```python
from build123d import *

# Parameters (mm, degrees)
SKETCH1_W           = 20.32
SKETCH1_H           = 134.62
BOSS_EXTRUDE1_DEPTH = 2.999994
BOSS_EXTRUDE2_DEPTH = 2.999994
BOSS_EXTRUDE3_DEPTH = 22.86
SKETCH4_R           = 2.54
CUT_EXTRUDE1_DEPTH  = 37.477194


with BuildPart() as part:
    # Sketch1 → Boss-Extrude1 (new body)
    with BuildSketch(Plane.XY):
        with Locations((-1.678928241, 0)):
            Rectangle(SKETCH1_W, SKETCH1_H)
    extrude(amount=BOSS_EXTRUDE1_DEPTH)

    # Sketch2 → Boss-Extrude2 (add)
    with BuildSketch(Plane(origin=(0, -67.31, 0), x_dir=(1, 0, 0), z_dir=(0, 1, 0))):
        Polygon((-11.838928241, 0), (-11.838928241, 16.7386), (8.478742997, 16.7386), (8.481071759, 0), (8.478742997, -2.999994), (8.481071759, -19.738594), (-11.838928241, -19.738594), (-11.838928241, -2.999994), align=None)
    extrude(amount=BOSS_EXTRUDE2_DEPTH)

    # Sketch3 → Boss-Extrude3 (add)
    with BuildSketch(Plane(origin=(0, -67.31, 0), x_dir=(-1, 0, 0), z_dir=(0, -1, 0))):
        Polygon((11.838928241, 16.7386), (11.838928241, 13.72362), (-8.479162457, 13.72362), (-8.478742997, 16.7386), align=None)
        Polygon((-8.481065309, -16.677248459), (-8.481065309, -19.692228459), (11.837025389, -19.692228459), (11.836605929, -16.677248459), align=None)
    extrude(amount=BOSS_EXTRUDE3_DEPTH)

    # Sketch4 → Cut-Extrude1 (cut, through all)
    with BuildSketch(Plane(origin=(0, 0, -16.7386), x_dir=(-1, 0, 0), z_dir=(0, 0, -1))):
        with Locations((1.680092622, -84.961272754)):
            Circle(SKETCH4_R)
    extrude(amount=-CUT_EXTRUDE1_DEPTH, mode=Mode.SUBTRACT)


solid = part.part
```
Design review of the part built by this model. Coordinates are the model's own, in mm. A direction names the side the tool comes from. Coordinates: 2 decimals unless noted, no trailing zeros. Order: outer loops, then holes, each group sorted by start corner. A loop starts at its lowest first (then second) coordinate and runs counter-clockwise, first axis right, second up.
1) Take a section at C-C, the plane x = -1.5. Give the boundary of the cut face in (y, z), and give its area (3 significant figures).
2) For faces 4 (the flat face through (-2, -79, -13.724)), 5 (the flat face through (-2, 1, 3)), 6 (the flat face through (-2, -77, -16.739)), 7 (the flat face through (-2, -64.31, -8)), list the 3-axis set-ups (+Z, -Z, +X, -X, +Y, -Y) from which the entire face can be reached by the end or side of a thin tool; tool diameter is ignored.
3) Take a section at A-A, the plane y = -76. Give the boundary of the cut face in (x, z).
4) Clearance check with flat-ended pins moving along their axes: pin 1 (6.5 mm diameter, centred on x = -1.68, y = -84.96, fed in from -Z); pin 2 (1 mm diameter, centred on x = -8, z = -6, fed in from +Y); pin 3 (4 mm diameter, centred on x = -5.5, y = -36.5, fed in from -Z); pin 4 (4 mm diameter, centred on x = -4.5, z = 12.5, fed in from -Y). State where each tip first meets the part, or that it passes through.
5) Take a section at B-B, the plane x = -8.25. Give the boundary of the cut face in (y, z).
6) Take a section at D-D, the plane y = 22.5. Give the boundary of the cut face in (x, z), and give its area (3 significant figures).
7) Wall thickness on line 1 along Y through (x, z) = (4, 17); line 2 along Y through (x, z) = (-4, -10); line 3 along Z through (x, y) = (-10.5, -81.5): over which ranges is each line inside the solid? List them lowest first.
8) Mouldability with a two-part tool opening along Z and no side actions: class faces 1 (the flat face through (-2, -66, 19.739)), 2 (the flat face through (-2, -90.17, -15)), 3 (the flat face through (-2, -67.31, 3)) as +Z half, -Z half, draft (parallel to the pull), parting line (faces both ways), or undercut.
Returned:
1. outline: (-90.17, -16.74) - (-87.49, -16.74) - (-87.49, -13.72) - (-90.17, -13.72) - close; (-90.17, 16.68) - (-87.49, 16.68) - (-87.49, 19.69) - (-90.17, 19.69) - close; (-82.43, -16.74) - (-64.31, -16.74) - (-64.31, 0) - (67.31, 0) - (67.31, 3) - (-64.31, 3) - (-64.31, 19.74) - (-67.31, 19.74) - (-67.31, 19.69) - (-82.43, 19.69) - (-82.43, 16.68) - (-67.31, 16.68) - (-67.31, -13.72) - (-82.43, -13.72) - close
1. area: 612 mm2
2. face 4: +X, -X, -Y
2. face 5: +Z, +X, -X, +Y
2. face 6: -Z, +X, -X, +Y, -Y
2. face 7: -Z, +X, -X, +Y
3. outline: (-11.84, -16.74) - (8.48, -16.74) - (8.48, -13.72) - (-11.84, -13.72) - close; (-11.84, 16.68) - (8.48, 16.68) - (8.48, 19.69) - (-11.84, 19.69) - close
4. pin 1: stops at z = -16.74
4. pin 2: stops at y = -64.31
4. pin 3: stops at z = 0
4. pin 4: stops at y = -67.31
5. outline: (-90.17, -16.74) - (-64.31, -16.74) - (-64.31, 0) - (67.31, 0) - (67.31, 3) - (-64.31, 3) - (-64.31, 19.74) - (-67.31, 19.74) - (-67.31, 19.69) - (-90.17, 19.69) - (-90.17, 16.68) - (-67.31, 16.68) - (-67.31, -13.72) - (-90.17, -13.72) - close
6. outline: (-11.84, 0) - (8.48, 0) - (8.48, 3) - (-11.84, 3) - close
6. area: 61.0 mm2
7. line 1: y = -90.17 to -64.31
7. line 2: y = -67.31 to -64.31
7. line 3: z = -16.74 to -13.72, 16.68 to 19.69
8. face 1: +Z half
8. face 2: draft
8. face 3: undercut
